Can you work these out from the model? Positions are in its coordinate system, mm. Face numbers are marked on the shaded views. A direction names the side the tool comes from. Round coordinates to 2 decimals unless told otherwise and drop trailing zeros. Loops run counter-clockwise (first coordinate to the right, second up) from the corner with the lowest first, then second, coordinate; pieces in that order, holes last. Notation, with made-up numbers: (26, 85) -> (55, 85) arc R19 cw to (55, 113) -> close; hole circle Ø10 at (60, 38.5). An arc over 180 degrees is marked (long way). Write item = value, one per line.
from build123d import *

# Parameters (mm, degrees)
SKETCH2_W              = 4
SKETCH2_H              = 40
SKETCH2_W_2            = 9.675
SKETCH2_W_3            = 9.65
BOTTOMBASE_DEPTH       = 3.5
EXTRUDE_START          = 3.5
SKETCH2_3_W            = 9.675
SKETCH2_3_H            = 40
SKETCH2_3_W_2          = 4
EXTRUDE_U_DEPTH        = 9.8
TOPFORU_START          = 13.3
SKETCH2_5_W            = 37
SKETCH2_5_H            = 40
TOPFORU_DEPTH          = 3
ANGLEDBOTTOM_SIZE      = 8
ANGLEDBOTTOM_SIZE2     = 11.425184054
SIDESTOHOLDMOTOR_START = 16.3
SKETCH2_4_W            = 4
SKETCH2_4_H            = 40
SIDESTOHOLDMOTOR_DEPTH = 25
SKETCH3_W              = 33.690968993
SKETCH3_H              = 4
ZIPTIEHOLE_DEPTH       = 1.5
SKETCH4_W              = 50.344511624
SKETCH4_H              = 4
ZIPTIEHOLE2_DEPTH      = 1.5


with BuildPart() as part:
    # Sketch2 → BottomBase (new body)
    with BuildSketch(Plane.XY):
        with Locations((-16.5, 0)):
            Rectangle(SKETCH2_W, SKETCH2_H)
        with Locations((-9.6625, 0)):
            Rectangle(SKETCH2_W_2, SKETCH2_H)
        Rectangle(SKETCH2_W_3, SKETCH2_H)
        with Locations((9.6625, 0)):
            Rectangle(SKETCH2_W_2, SKETCH2_H)
        with Locations((16.5, 0)):
            Rectangle(SKETCH2_W, SKETCH2_H)
    extrude(amount=BOTTOMBASE_DEPTH)

    # Sketch2<3> → U (add)
    with BuildSketch(Plane.XY.offset(EXTRUDE_START)):
        with Locations((9.6625, 0)):
            Rectangle(SKETCH2_3_W, SKETCH2_3_H)
        with Locations((16.5, 0)):
            Rectangle(SKETCH2_3_W_2, SKETCH2_3_H)
        with Locations((-9.6625, 0)):
            Rectangle(SKETCH2_3_W, SKETCH2_3_H)
        with Locations((-16.5, 0)):
            Rectangle(SKETCH2_3_W_2, SKETCH2_3_H)
    extrude(amount=EXTRUDE_U_DEPTH)

    # Sketch2<5> → topForU (add)
    with BuildSketch(Plane.XY.offset(TOPFORU_START)):
        Rectangle(SKETCH2_5_W, SKETCH2_5_H)
    extrude(amount=TOPFORU_DEPTH)

    # angledBottom
    angledbottom_edges = [part.edges().sort_by_distance(p)[0] for p in [
        (18.5, 0, 0),
        (-18.5, 0, 0),
    ]]
    angledbottom_side = [part.faces().sort_by_distance(p)[0] for p in [
        (0, 0, 0),
    ]]
    chamfer(angledbottom_edges, length=ANGLEDBOTTOM_SIZE, length2=ANGLEDBOTTOM_SIZE2, reference=angledbottom_side[0])

    # Sketch2<4> → sidesToHoldMotor (add)
    with BuildSketch(Plane.XY.offset(SIDESTOHOLDMOTOR_START)):
        with Locations((-16.5, 0)):
            Rectangle(SKETCH2_4_W, SKETCH2_4_H)
        with Locations((16.5, 0)):
            Rectangle(SKETCH2_4_W, SKETCH2_4_H)
    extrude(amount=SIDESTOHOLDMOTOR_DEPTH)

    # Sketch3 → zipTieHole (cut)
    with BuildSketch(Plane(origin=(7.045605752, 0, -4.933386259), x_dir=(-0.5735764363510474, 0, -0.819152044288991), z_dir=(0.819152044288991, 0, -0.5735764363510474))):
        with Locations((-9.106215993, 0)):
            Rectangle(SKETCH3_W, SKETCH3_H)
        with Locations((-9.106215993, 14)):
            Rectangle(SKETCH3_W, SKETCH3_H)
        with Locations((-9.106215993, -14)):
            Rectangle(SKETCH3_W, SKETCH3_H)
    extrude(amount=-ZIPTIEHOLE_DEPTH, mode=Mode.SUBTRACT)

    # Sketch4 → zipTieHole2 (cut)
    with BuildSketch(Plane(origin=(-7.045605752, 0, -4.933386259), x_dir=(-0.5735764363510474, 0, 0.819152044288991), z_dir=(-0.819152044288991, 0, -0.5735764363510474))):
        Rectangle(SKETCH4_W, SKETCH4_H)
        with Locations((0, 14)):
            Rectangle(SKETCH4_W, SKETCH4_H)
        with Locations((0, -14)):
            Rectangle(SKETCH4_W, SKETCH4_H)
    extrude(amount=-ZIPTIEHOLE2_DEPTH, mode=Mode.SUBTRACT)


solid = part.part
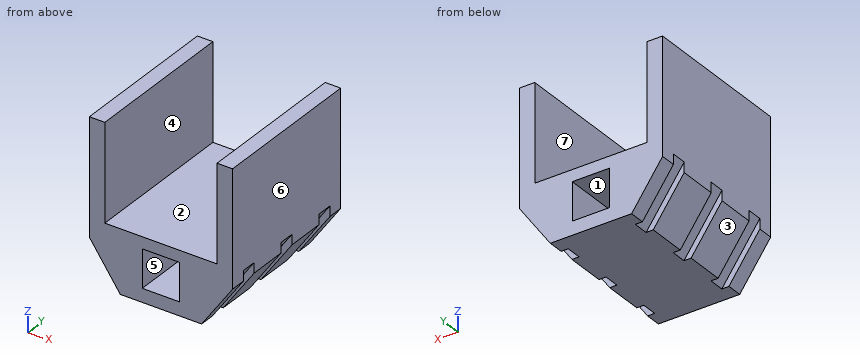
1. Suppose I cut it at B-B, the plane y = -9. List the corners of the cut face in (x, z) for me (3 decimals), and give its area (3 significant figures).
Entries:
outline = (-18.5, 11.425) -> (-10.5, 0) -> (10.5, 0) -> (18.5, 11.425) -> (18.5, 41.3) -> (14.5, 41.3) -> (14.5, 16.3) -> (-14.5, 16.3) -> (-14.5, 41.3) -> (-18.5, 41.3) -> close; hole (-4.825, 3.5) -> (4.825, 3.5) -> (4.825, 13.3) -> (-4.825, 13.3) -> close
area = 617 mm²
2. For the marked faces 5, 6 and 7, which set-ups out of +Z, -Z, +X, -X, +Y, -Y let a thin tool reach every point of the face, with its end or its side?
Entries:
face_5 = +Y, -Y
face_6 = +Z, -Z, +X, +Y, -Y
face_7 = +Z, +Y, -Y
3. I need wall thicknesses on line 1 (X direction, y = -17, z = 17); line 2 (Z direction, x = 0, y = 6); line 3 (X direction, y = -17, z = 12) (3 decimals). Which ranges of each line are inside material? Lowest first, please. Write a range as [from, to].
Entries:
line_1 = [-18.5, -14.5], [14.5, 18.5]
line_2 = [0, 3.5], [13.3, 16.3]
line_3 = [-18.5, -4.825], [4.825, 18.5]
4. We'd pull the mould along Z, two halves only. Please class the marked faces 1, 2, 3 and 4: released by +Z, released by -Z, zero draft, split by the parting line, or undercut.
Entries:
face_1 = undercut
face_2 = released by +Z
face_3 = released by -Z
face_4 = zero draft
5. Suppose I cut it at A-A, the plane z = 27.5. List the corners of the cut face in (x, y) for me, and give its area (3 significant figures).
Entries:
outline = (-18.5, -20) -> (-14.5, -20) -> (-14.5, 20) -> (-18.5, 20) -> close; (14.5, -20) -> (18.5, -20) -> (18.5, 20) -> (14.5, 20) -> close
area = 320 mm²
6. Suppose I cut it at D-D, the plane y = 0.5. List the corners of the cut face in (x, z) for me (3 decimals).
Entries:
outline = (-18.5, 14.04) -> (-8.669, 0) -> (8.669, 0) -> (18.5, 14.04) -> (18.5, 41.3) -> (14.5, 41.3) -> (14.5, 16.3) -> (-14.5, 16.3) -> (-14.5, 41.3) -> (-18.5, 41.3) -> close; hole (-4.825, 3.5) -> (4.825, 3.5) -> (4.825, 13.3) -> (-4.825, 13.3) -> close
7. I'm going to push flat-ended pins straight in: pin 1 (3 mm diameter, centred on y = 7.5, z = 7.5, fed in from -X); pin 2 (1.5 mm diameter, centred on x = -14.5, y = -2.5, fed in from -Z); pin 3 (8.5 mm diameter, centred on x = -1, y = 0, fed in from +Z). Where does each tip first touch, or does it pass through?
Entries:
pin_1 = -16.8
pin_2 = 4.64
pin_3 = 16.3
8. Suppose I cut it at C-C, the plane x = 3. List the corners of the cut face in (y, z) for me, and give its area (3 significant figures).
Entries:
outline = (-20, 0) -> (20, 0) -> (20, 3.5) -> (-20, 3.5) -> close; (-20, 13.3) -> (20, 13.3) -> (20, 16.3) -> (-20, 16.3) -> close
area = 260 mm²
